Autodesk Inventor part; units mm, degrees
ref_plane "YZ Plane" through (0, 0, 0) normal (1, 0, 0) x (0, 1, 0)
ref_plane "XZ Plane" through (0, 0, 0) normal (0, 1, 0) x (-1, 0, 0)
ref_plane "XY Plane" through (0, 0, 0) normal (0, 0, 1) x (1, 0, 0)
sketch "Sketch1" plane through (0, 0, 0) normal (0, 0, 1) x (1, 0, 0)
  line L0 (0, 0) -> (25.4, 0)
  line L1 (25.4, 0) -> (25.4, 25.4)
  line L2 (25.4, 25.4) -> (0, 25.4)
  line L3 (0, 25.4) -> (0, 0)
  line L4 (3.175, 22.225) -> (22.225, 22.225)
  line L5 (22.225, 22.225) -> (22.225, 3.175)
  line L6 (22.225, 3.175) -> (3.175, 3.175)
  line L7 (3.175, 3.175) -> (3.175, 22.225)
  dimension "d0" = 25.4
  dimension "d1" = 25.4
  dimension "d2" = 3.175
extrude "Extrusion1" add sketch "Sketch1" against normal blind 355.6
sketch "Sketch2" plane through (0, 0, 0) normal (-1, 0, 0) x (0, 0, 1)
  line L0 (0, 25.4) -> (-355.6, 25.4)
  line L1 (0, 25.4) -> (0, 0)
  point P0 (-317.5, 12.7)
  point P1 (-292.1, 12.7)
  point P2 (-12.7, 12.7)
  point P3 (-38.1, 12.7)
  point P4 (-63.5, 12.7)
  point P5 (-317.5, 12.7)
  point P6 (-342.9, 12.7)
  dimension "d6" = 25.4
  dimension "d7" = 12.7
  dimension "d24" = 12.7
  dimension "d25" = 25.4
  dimension "d26" = 25.4
  dimension "d27" = 25.4
  dimension "d31" = 25.4
  dimension "d32" = 228.6
hole "Hole1" at (0, 12.7, -317.5) at (0, 12.7, -292.1) at (0, 12.7, -38.1) at (0, 12.7, -12.7) at (0, 12.7, -63.5) at (0, 12.7, -342.9) direction (1, 0, 0) diameter 6.35 depth 25.4 tip angle 118
sketch "Sketch5" plane through (0, 25.4, 0) normal (0, 1, 0) x (1, 0, 0)
  line L0 (25.4, 0) -> (0, 0)
  point P0 (12.7, 152.4)
  dimension "d34" = 152.4
hole "Hole3" at (12.7, 25.4, -152.4) direction (0, -1, 0) diameter 6.35 depth 25.4 tip angle 118
properties part number "towermiddleunderthing"
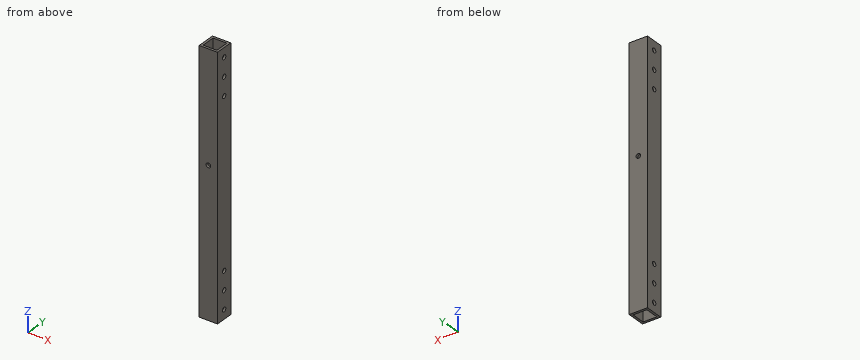
Input: part model. Units: mm. Frame: model coordinates. Round coordinates to 2 decimals unless told otherwise and drop trailing zeros. Order: outer loops, then holes, each group sorted by start corner. A loop starts at its lowest first (then second) coordinate and runs counter-clockwise, first axis right, second up.
1. Cut plane B-B, the plane z = -38.1. Output: boundary loops of the cut face in (x, y) (3 decimals).
The answers:
outline: (0, 0) - (25.4, 0) - (25.4, 9.525) - (22.225, 9.525) - (22.225, 3.175) - (3.175, 3.175) - (3.175, 9.525) - (0, 9.525) - close; (0, 15.875) - (3.175, 15.875) - (3.175, 22.225) - (22.225, 22.225) - (22.225, 15.875) - (25.4, 15.875) - (25.4, 25.4) - (0, 25.4) - close
2. Cut plane C-C, the plane x = 12.7. Output: boundary loops of the cut face in (y, z) (3 decimals), then the cut area to 3 significant figures.
The answers:
outline: (0, -355.6) - (3.175, -355.6) - (3.175, -155.575) - (0, -155.575) - close; (0, -149.225) - (3.175, -149.225) - (3.175, 0) - (0, 0) - close; (22.225, -355.6) - (25.4, -355.6) - (25.4, -155.575) - (22.225, -155.575) - close; (22.225, -149.225) - (25.4, -149.225) - (25.4, 0) - (22.225, 0) - close
area: 2,220 mm2
3. Material intervals for line 1 (Y direction, x = 1, z = -292.1) (3 decimals); line 2 (X direction, y = 5.5, z = -132) (3 decimals), sorted ascending.
The answers:
line 1: y = 0 to 9.525, 15.875 to 25.4
line 2: x = 0 to 3.175, 22.225 to 25.4
4. Cut plane A-A, the plane y = 19. Output: boundary loops of the cut face in (x, z) (3 decimals), then the cut area to 3 significant figures.
The answers:
outline: (0, -355.6) - (3.175, -355.6) - (3.175, 0) - (0, 0) - close; (22.225, -355.6) - (25.4, -355.6) - (25.4, 0) - (22.225, 0) - close
area: 2,260 mm2
5. Cut plane D-D, the plane z = -177. Output: boundary loops of the cut face in (x, y) (3 decimals), then the cut area to 3 significant figures.
The answers:
outline: (0, 0) - (25.4, 0) - (25.4, 25.4) - (0, 25.4) - close; hole (3.175, 3.175) - (22.225, 3.175) - (22.225, 22.225) - (3.175, 22.225) - close
area: 282 mm2
